Could you check a few things on this drawing? It's one solid part, dimensions in mm from its lowest x, y, z. Coordinates: 2 decimals unless noted, no trailing zeros. Loops run counter-clockwise (first coordinate to the right, second up) from the corner with the lowest first, then second, coordinate; pieces in that order, holes last. Notation, with made-up numbers: (67.5, 48) -> (90.5, 48) arc R25 ccw to (90.5, 85) -> close; hole circle Ø3 at (3.25, 44.25). An arc over 180 degrees is marked (long way). One line per question, with ' | ' between items. Start each with the question number.
(1) Suppose I cut it at A-A (x = 12.25). Please give me the cut outline in (y, z) (3 decimals).
(2) Suppose I cut it at C-C (x = 8.5). Please give me the cut outline in (y, z) (3 decimals).
(3) If I drill on line 1 along X through (y, z) = (7.75, 5.25); line 2 along X through (y, z) = (4.5, 2); line 3 along Z through (x, y) = (6.5, 5.75), over which ranges is the centre line in solid material (lowest first)?
(4) I'm going to push flat-ended pins straight in: pin 1 Ø5 at (x, y) = (6, 7.5) entering from -Z; pin 2 Ø1.5 at (x, z) = (5, 6.5) entering from +Y. Where does each tip first touch, or does it pass through?
(5) Suppose I cut it at B-B (x = 16.5). Please give me the cut outline in (y, z) (3 decimals).
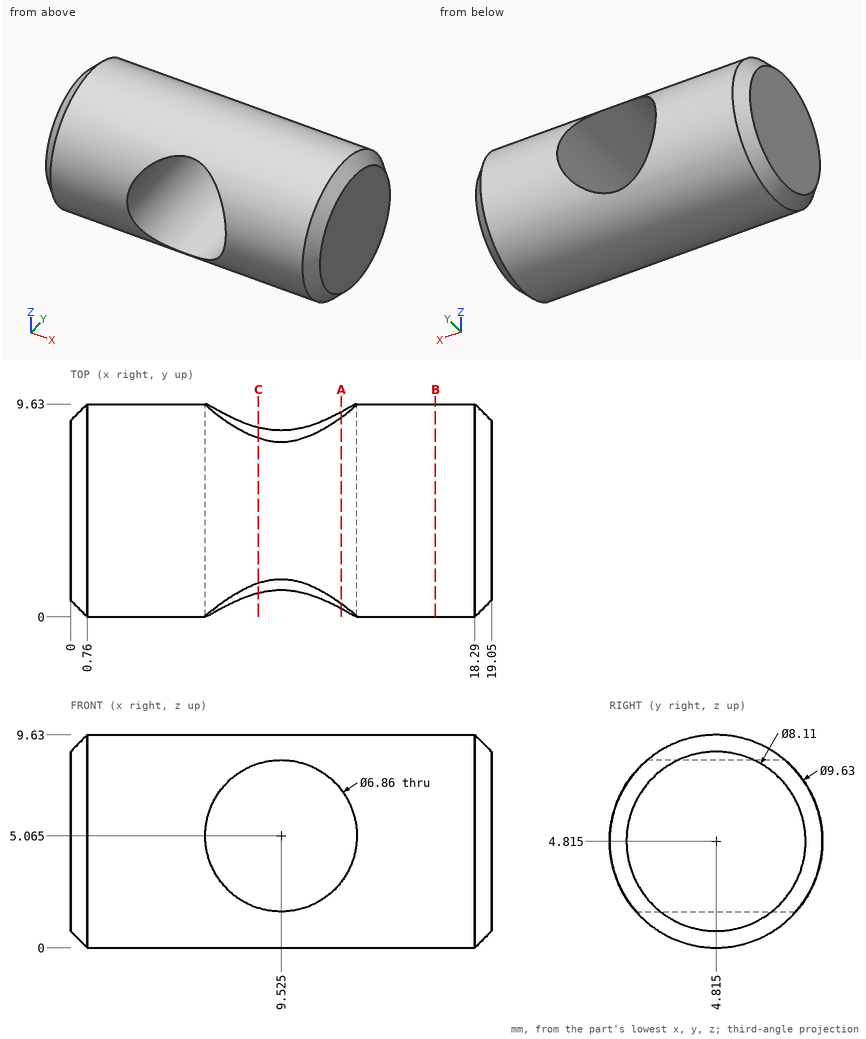
Checks:
1) outline: (0.363, 2.982) arc R4.815 ccw to (9.267, 2.982) -> close; (0.603, 7.148) -> (9.027, 7.148) arc R4.815 ccw to start
2) outline: (1.067, 1.792) arc R4.815 ccw to (8.563, 1.792) -> close; (1.533, 8.338) -> (8.097, 8.338) arc R4.815 ccw to start
3) line 1: x = 0 to 6.1, 12.95 to 19.05 | line 2: x = 0 to 7.99, 11.06 to 19.05 | line 3: z = 0.09 to 3.45, 6.68 to 9.54
4) pin 1: stops at z = 0 | pin 2: stops at y = 9.54
5) outline: circle Ø9.63 at (4.815, 4.815)
